The model under review builds one solid part; all positions refer to its coordinate system, in mm. Round coordinates to 2 decimals unless told otherwise and drop trailing zeros. Write each loop counter-clockwise with the first axis right and the second up, starting at its lowest first coordinate (ties: lowest second). Pieces come first, ordered by that corner, then holes.
Item 1: Clearance check with flat-ended pins moving along their axes: pin 1 Ø2 at (y, z) = (-2, 3.5) entering from +X; pin 2 Ø1 at (x, y) = (6, -4) entering from +Z; pin 3 Ø1 at (y, z) = (-4.5, 1) entering from +X; pin 4 Ø1 at (x, z) = (-3.5, 1) entering from +Y. State where each tip first meets the part, or that it passes through.
Item 2: To check wall thickness, follow L1, parallel to X at y = -8, z = 4; L2, parallel to X at y = -8.5, z = 2; L3, parallel to Z at x = 7.75, y = -6. State the ranges of each line that lie inside material, in increasing order.
Item 3: Add section D-D (x = 3.75). Give the boundary of the cut face in (y, z).
Item 4: Add section B-B (y = -8.25). Give the boundary of the cut face in (x, z).
Item 5: Add section C-C (x = 0). Give the boundary of the cut face in (y, z).
Item 6: Add section A-A (z = 5.25). Give the boundary of the cut face in (x, y).
```python
from build123d import *

# Parameters (mm, degrees)
F0_R     = 9
F0_R_2   = 5.65
F1_DEPTH = 9
F3_DEPTH = 25
F5_DEPTH = 25


with BuildPart() as f1:
    # F0 (on Front) → F1 (new body)
    with BuildSketch(Plane.XZ):
        Circle(F0_R)
        Circle(F0_R_2, mode=Mode.SUBTRACT)
    extrude(amount=F1_DEPTH)

    # F2 (on face) → F3 (cut)
    with BuildSketch(Plane.XZ.offset(9)):
        Polygon((9.609743, 0), (-9, 0), (-9.972616, 0), (-9.972616, -10.801357), (9.609743, -10.801357), align=None)
    extrude(amount=-F3_DEPTH, mode=Mode.SUBTRACT)

    # F4 (on face) → F5 (cut)
    with BuildSketch(Plane.XZ.offset(9)):
        Polygon((-7.133957, 7.65), (0, 7.65), (5.867002, 7.65), (5.867002, 11.901876), (-7.133957, 11.901876), align=None)
    extrude(amount=-F5_DEPTH, mode=Mode.SUBTRACT)


solid = f1.part
```
Numbers:
1. pin 1: stops at x = 8.65
1. pin 2: stops at z = 7.12
1. pin 3: stops at x = 8.99
1. pin 4: passes through
2. L1: x = -8.06 to -3.99, 3.99 to 8.06
2. L2: x = -8.77 to -5.28, 5.28 to 8.77
2. L3: z = 0 to 4.58
3. outline: (-9, 4.23) - (0, 4.23) - (0, 7.65) - (-9, 7.65) - close
4. outline: (-9, 0) - (-5.65, 0) arc R5.65 cw to (5.65, 0) - (9, 0) arc R9 ccw to (4.74, 7.65) - (-4.74, 7.65) arc R9 ccw to start
5. outline: (-9, 5.65) - (0, 5.65) - (0, 7.65) - (-9, 7.65) - close
6. outline: (-7.31, -9) - (-2.09, -9) - (-2.09, 0) - (-7.31, 0) - close; (2.09, -9) - (7.31, -9) - (7.31, 0) - (2.09, 0) - close
